from build123d import *

# Parameters (mm, degrees)
SKETCH1_R           = 4.8
BOSS_EXTRUDE1_DEPTH = 15
CUT_EXTRUDE1_DEPTH  = 1


with BuildPart() as part:
    # Sketch1 → Boss-Extrude1 (new body)
    with BuildSketch(Plane(origin=(0, 0, 0), x_dir=(1, 0, 0), z_dir=(0, 1, 0))):
        with Locations(Location((0, 0, 0), (0, 0, 270))):  # turned: the seam where the file's is
            Circle(SKETCH1_R)
    extrude(amount=BOSS_EXTRUDE1_DEPTH)

    # Sketch2 → Cut-Extrude1 (cut, symmetric)
    with BuildSketch(Plane(origin=(0, 0, 0), x_dir=(0, 0, -1), z_dir=(1, 0, 0))):
        Polygon((-2.5, 0), (2.5, 0), (2.5, 4), (2, 4), (2, 8), (-2, 8), (-2, 4), (-2.5, 4), align=None)
    extrude(amount=CUT_EXTRUDE1_DEPTH, both=True, mode=Mode.SUBTRACT)


solid = part.part
The listing builds one solid part. Answer for the finished solid, in the listing's coordinates (mm). A direction names the side the tool comes from. Give positions to 0.01 mm unless a question says otherwise; leave off trailing zeros. Loops run counter-clockwise (first coordinate to the right, second up) from the corner with the lowest first, then second, coordinate; pieces in that order, holes last. Notation, with made-up numbers: (3.5, 50) - (26.5, 50) arc R10 ccw to (26.5, 64) - close; hole circle Ø7 at (18.25, -38.75). An arc over 180 degrees is marked (long way). Use one line per item in the form item = value.
1. Section C-C on z = 0 is taken. Give the vertices of the cut face in (x, y), then the cut area to 3 significant figures.
Calculated:
outline = (-4.8, 0) - (-1, 0) - (-1, 8) - (1, 8) - (1, 0) - (4.8, 0) - (4.8, 15) - (-4.8, 15) - close
area = 128 mm^2
2. Section D-D on y = 9 is taken. Give the vertices of the cut face in (x, z).
Calculated:
outline = circle Ø9.6 at (0, 0)
3. Section B-B on x = 0 is taken. Give the vertices of the cut face in (y, z), then the cut area to 3 significant figures.
Calculated:
outline = (0, -4.8) - (15, -4.8) - (15, 4.8) - (0, 4.8) - (0, 2.5) - (4, 2.5) - (4, 2) - (8, 2) - (8, -2) - (4, -2) - (4, -2.5) - (0, -2.5) - close
area = 108 mm^2
4. Given pin 1 Ø1.6 at (x, z) = (0, -0.5) entering from -Y, flat-ended and moving along its own axis, determine where the tip first touches the part or whether it passes through.
Calculated:
pin_1 = 8
5. Find the intervals of material crossed by line 1 along X through (y, z) = (6.25, 1.25); line 2 along Y through (x, z) = (-0.75, 1.5); line 3 along X through (y, z) = (7, -3), in increasing order. Write a range as [from, to].
Calculated:
line_1 = [-4.63, -1], [1, 4.63]
line_2 = [8, 15]
line_3 = [-3.75, 3.75]
6. Which of the six approach directions +Z, -Z, +X, -X, +Y, -Y give full straight-line access (tool end or side, diameter ignored) to faces 4 (the face through (0, 15, 0)), 5 (the face through (0, 2, 2.5))?
Calculated:
face_4 = +Z, -Z, +X, -X, +Y
face_5 = -Y
7. The mould has two halves that part along X. Classify faces 1 (the face through (-1, 4, 0)), 2 (the face through (-2, 0, 0)), 3 (the face through (4.05, 7.4, 2.58)): pulls with the +X half, pulls with the -X half, needs draft (parallel to the pull), parting line crosses it, or undercut.
Calculated:
face_1 = undercut
face_2 = needs draft
face_3 = parting line crosses it
8. Section A-A on y = 2.25 is taken. Give the vertices of the cut face in (x, z).
Calculated:
outline = circle Ø9.6 at (0, 0); hole (-1, -2.5) - (1, -2.5) - (1, 2.5) - (-1, 2.5) - close
